Check sheet for the modelled part. Datum: model origin and axes. Units: mm. A direction names the side the tool comes from. Coordinates: 2 decimals unless noted, no trailing zeros. Write each loop counter-clockwise with the first axis right and the second up, starting at its lowest first coordinate (ties: lowest second). Pieces come first, ordered by that corner, then holes. Notation, with made-up numbers: (51.25, 43) -> (70.25, 43) arc R22 cw to (70.25, 59) -> close; hole circle Ø1 at (-12, -26). An arc over 180 degrees is marked (long way). One line per item, written item: value. Start each with the question number.
1) Draft check along Z on faces 3 (the conical face through (-58.823, 11.6, 45.104)), 4 (the cylindrical face through (-65.32, 6.01, -2.49)), 5 (the flat face through (-1, 12.192, 15)). Enter one of: +Z half, -Z half, draft (parallel to the pull), parting line (faces both ways), or undercut.
2) Gauge pin test, flat ends, axial feed: P1, Ø12.5, axis at x = 41.08, z = 44.45, coming from the -Y side; P2, Ø6, axis at x = -45.5, y = 6.5, coming from the +Z side; P3, Ø3, axis at y = 3.5, z = -8.5, coming from the -X side; P4, Ø2, axis at x = -25.5, y = 10.5, coming from the +Z side. Record the tip position at first contact, or that the pin passes through.
3) Set-up check for faces 1 (the cylindrical face through (44.9, 9.6, -41.6)), 2 (the cylindrical face through (65.985, 6.011, 1.284)): record each of +Z, -Z, +X, -X, +Y, -Y from which the full face is reachable in a straight line by a thin tool's end or side.
4) Sectioned sample at A-A on x = 0. Enter the section's corners in (y, z) (3 decimals), plus the area to 3 significant figures.
5) Sectioned sample at B-B on y = 9.5. Give the number of separate pieces and of enclosed holes in the cut face, plus the area to 3 significant figures.
6) Scan lines: line 1 along X through (y, z) = (11.15, -44.45); line 2 along X through (y, z) = (10.25, 44); line 3 along X through (y, z) = (11.5, -2). Record each from-to range of solid material in increasing order. Write a range as [from, to].
```python
from build123d import *

# Parameters (mm, degrees)
SKETCH1_R                        = 85.725
BOSS_EXTRUDE1_DEPTH              = 12.192
BOSS_EXTRUDE1_TAPER              = 45
F_3_8_16_TAPPED_HOLE1_D          = 7.9375
F_1_4_0_25_PRESS_DOWEL_HOLE1_D   = 6.35
F_3_8_0_375_DIAMETER_HOLE1_D     = 9.525
F_3_8_0_375_DIAMETER_HOLE1_DEPTH = 5.08
F_3_8_0_375_DIAMETER_HOLE1_TIP   = 2.861598698


with BuildPart() as part:
    # Sketch1 → Boss-Extrude1 (new body)
    with BuildSketch(Plane(origin=(0, 0, 0), x_dir=(1, 0, 0), z_dir=(0, 1, 0))):
        Circle(SKETCH1_R)
    extrude(amount=BOSS_EXTRUDE1_DEPTH, taper=BOSS_EXTRUDE1_TAPER)

    # 3/8-16 Tapped Hole1 (through all)
    with Locations(Plane(origin=(0, 12.192, 0), x_dir=(-0.9997060077974085, 0, -0.024246607469250836), z_dir=(0, 1, 0))):
        with Locations((62.211704865, 1.508866383), (-62.211704865, -1.508866383)):
            Hole(F_3_8_16_TAPPED_HOLE1_D / 2)

    # 1/4 (0.25) Press Dowel Hole1 (through all)
    with Locations(Plane(origin=(-177.991498203, 12.192, 193.466008664), x_dir=(-0.909586317376337, 0, -0.4155150192733753), z_dir=(0, 1, 0))):
        with Locations((-81.510599056, -249.932175164)):
            Hole(F_1_4_0_25_PRESS_DOWEL_HOLE1_D / 2)

    # 3/8 (0.375) Diameter Hole1
    with Locations(Plane(origin=(0, 12.192, 0), x_dir=(1, 0, 0), z_dir=(0, 1, 0))):
        with Locations((-41.0845, 44.45), (-41.0845, 0), (-41.0845, -44.45), (41.0845, -44.45), (41.0845, 0), (41.0845, 44.45)):
            Hole(F_3_8_0_375_DIAMETER_HOLE1_D / 2, depth=F_3_8_0_375_DIAMETER_HOLE1_DEPTH)
            with Locations((0, 0, -(F_3_8_0_375_DIAMETER_HOLE1_DEPTH + F_3_8_0_375_DIAMETER_HOLE1_TIP / 2))):  # 118° drill point
                Cone(0, F_3_8_0_375_DIAMETER_HOLE1_D / 2, F_3_8_0_375_DIAMETER_HOLE1_TIP, mode=Mode.SUBTRACT)


solid = part.part
```
Answers:
1. face 3: parting line
1. face 4: undercut
1. face 5: draft
2. P1: stops at y = 0
2. P2: stops at z = 68.99
2. P3: stops at x = -83.3
2. P4: stops at z = 71.89
3. face 1: +Y
3. face 2: +Y, -Y
4. outline: (0, -85.725) -> (12.192, -73.533) -> (12.192, -3.175) -> (0, -3.175) -> close; (0, 3.175) -> (12.192, 3.175) -> (12.192, 73.533) -> (0, 85.725) -> close
4. area: 1,860 mm2
5. separate pieces: 1
5. enclosed holes: 9
5. area: 17,700 mm2
6. line 1: x = [-59.88, -45.85], [-36.32, 36.32], [45.85, 59.88]
6. line 2: x = [-61.32, -45.83], [-36.34, 36.34], [45.83, 61.32]
6. line 3: x = [-74.2, -65.66], [-58.8, -45.41], [-36.76, -2.47], [2.47, 36.76], [45.41, 58.8], [65.66, 74.2]
